```python
from build123d import *

# Parameters (mm, degrees)
F0_R       = 4
F1_DEPTH   = 15
F1_FACE1_R = 4
F3_DEPTH   = 15.001
F5_DEPTH   = 15


# Not quite as in the source:
# - a feature of the source that left no trace in its solid (it failed there, or was rolled back) is left out


with BuildPart() as f1:
    # F0 (on Top) → F1 (new body)
    with BuildSketch(Plane.XY):
        Polygon((5.5, -3.1754264805), (5.5, 3.1754264805), (0, 6.3508529611), (-5.5, 3.1754264805), (-5.5, -3.1754264805), (0, -6.3508529611), align=None)
        Circle(F0_R, mode=Mode.SUBTRACT)
    extrude(amount=F1_DEPTH)

    # F2 (on face) + F1_face1 (on face) → F3 (cut, through all)
    with BuildSketch(Plane.XY.offset(15)):
        with BuildLine():
            Line((-3.3567126222, 2.1754264805), (-5.5, 2.1754264805))
            Line((-5.5, 2.1754264805), (-5.5, -2.1754264805))
            Line((-5.5, -2.1754264805), (-3.3567126222, -2.1754264805))
            ThreePointArc((-3.3567126222, -2.1754264805), (-4, 0), (-3.3567126222, 2.1754264805))
        make_face()
    with BuildSketch(Plane(origin=(0, 0, 0), x_dir=(1, 0, 0), z_dir=(0, 0, -1))):
        Polygon((5.5, -3.1754264805), (5.5, 3.1754264805), (0, 6.3508529611), (-5.5, 3.1754264805), (-5.5, -3.1754264805), (0, -6.3508529611), align=None)
        Circle(F1_FACE1_R, mode=Mode.SUBTRACT)
    extrude(amount=-F3_DEPTH, dir=(0, 0, 1), mode=Mode.SUBTRACT)

    # F4 (on Top) → F5 (join, through all)
    with BuildSketch(Plane.XY):
        with BuildLine():
            add(Edge.make_bspline(
                [(-3.3567126222, 2.1754264805), (-3.3567126222, 1.5), (-4.7243783011, 1.2322496152), (-5.2691254391, 1.1014623302), (-6.9790180063, 0), (-5.2691254391, -1.1014623302), (-4.7243783011, -1.2322496152), (-3.3567126222, -1.5), (-3.3567126222, -2.1754264805)],
                knots=[0, 0, 0, 0, 0.1875096718, 0.3211964826, 0.5, 0.6788035174, 0.8124903282, 1, 1, 1, 1], degree=3))
            Line((-3.3567126222, 2.1754264805), (-5.5, 2.1754264805))
            add(Edge.make_bspline(
                [(-5.5, 2.1754264805), (-5.5, 1.5), (-6.8295402039, 1.2640494778), (-7.2493526274, 1.0792890587), (-8.0427649595, -0.000100502), (-7.2510852775, -1.0789459234), (-6.8212907124, -1.2661384452), (-5.5, -1.5), (-5.5, -2.2451365801)],
                knots=[0, 0, 0, 0, 0.2037356069, 0.3258802228, 0.4986187951, 0.6713573674, 0.7935019833, 1, 1, 1, 1], degree=3))
            Line((-5.5, -2.2451365801), (-3.3567126222, -2.1754264805))
        make_face()
    extrude(amount=F5_DEPTH)


solid = f1.part
```
The model under review builds one solid part; all positions refer to its coordinate system, in mm. A direction names the side the tool comes from. Give positions to 0.01 mm unless a question says otherwise; leave off trailing zeros. Write each loop counter-clockwise with the first axis right and the second up, starting at its lowest first coordinate (ties: lowest second). Pieces come first, ordered by that corner, then holes. Notation, with made-up numbers: (39.25, 83.5) - (52.25, 83.5) arc R26 ccw to (52.25, 101.5) - close; hole circle Ø2 at (-14.5, 60). An arc over 180 degrees is marked (long way). Answer in a Markdown table with one row per item. Add a question column.
1. We need section C-C on y = -5. Write out the cut boundary in (x, z).
2. We need section D-D on x = 4.25. Write out the cut boundary in (y, z), then the cut area to 3 significant figures.
3. We need section A-A on x = -0.5. Write out the cut boundary in (y, z).
4. Tool access review of faces 5 (the flat face through (-5.5, -3, 7)), 6 (the flat face through (-5.5, 3, 7)), 7 (the flat face through (5.5, 0, 7)): name each direction out of +Z, -Z, +X, -X, +Y, -Y from which nothing blocks a thin tool from reaching the whole face with its end or side.
5. We need section B-B on y = -2.75. Write out the cut boundary in (x, z), then the cut area to 3 significant figures.
6. Wall thickness on line 1 along X through (y, z) = (0, 7); line 2 along Y through (x, z) = (3, 13); line 3 along Y through (x, z) = (-1, 13.75): over which ranges is each line inside the solid? List them lowest first. Write a range as [from, to].
7. Draft analysis for pull direction X (two halves, no side actions). For faces 1 (the flat face through (2.712, -4.785, 7.395)), 2 (the cylindrical face through (4, 0, 7)), 3 (the flat face through (-2.712, 4.785, 7.395)), 4 (the flat face through (-4, -2, 0)), state which applies: +X half, -X half, draft (parallel to the pull), parting line (faces both ways), or undercut.
8. Insertion check: P1, Ø6.5, axis at x = 0, y = 0, coming from the -Z side; P2, Ø0.7, axis at y = -2.5, z = 9.5, coming from the -X side; P3, Ø5, axis at x = -3, z = 6.5, coming from the -Y side. Each pin has a flat end and moves straight along its axis. Give the tip position at first contact, or say it passes through.
Ans:
| question | item | result |
|---|---|---|
| 1 | outline | (-2.34, 0) - (2.34, 0) - (2.34, 15) - (-2.34, 15) - close |
| 2 | outline | (-3.9, 0) - (3.9, 0) - (3.9, 15) - (-3.9, 15) - close |
| 2 | area | 117 mm^2 |
| 3 | outline | (-6.06, 0) - (-3.97, 0) - (-3.97, 15) - (-6.06, 15) - close; (3.97, 0) - (6.06, 0) - (6.06, 15) - (3.97, 15) - close |
| 4 | face 5 | +Z, -Z, -X, -Y |
| 4 | face 6 | +Z, -Z, -X, +Y |
| 4 | face 7 | +Z, -Z, +X, +Y, -Y |
| 5 | outline | (-5.5, 0) - (-2.9, 0) - (-2.9, 15) - (-5.5, 15) - close; (2.9, 0) - (5.5, 0) - (5.5, 15) - (2.9, 15) - close |
| 5 | area | 77.9 mm^2 |
| 6 | line 1 | x = [-7.75, -6.36], [4, 5.5] |
| 6 | line 2 | y = [-4.62, -2.65], [2.65, 4.62] |
| 6 | line 3 | y = [-5.77, -3.87], [3.87, 5.77] |
| 7 | face 1 | +X half |
| 7 | face 2 | undercut |
| 7 | face 3 | -X half |
| 7 | face 4 | draft |
| 8 | P1 | passes through |
| 8 | P2 | stops at x = -5.5 |
| 8 | P3 | stops at y = -6.06 |
